```python
from build123d import *

# Parameters (mm, degrees)
SKETCH1_R                        = 39.7891
SKETCH1_R_2                      = 38.1635
BOSS_EXTRUDE1_DEPTH              = 411.48
CUT_EXTRUDE1_START               = -1.66704
SKETCH2_R                        = 1.778
CUT_EXTRUDE1_DEPTH               = 1.66704
CIRPATTERN1_COUNT                = 3
PRESSURE_START                   = -1.699963
SKETCH3_R                        = 2.38125
PRESSURE_EQUALIZATION_HOLE_DEPTH = 1.699963
CIRPATTERN2_COUNT                = 3
SKETCH4_R                        = 1.7859375
CUT_EXTRUDE3_DEPTH               = 1.667411
CIRPATTERN3_COUNT                = 3


with BuildPart() as part:
    # Sketch1 → Boss-Extrude1 (new body)
    with BuildSketch(Plane(origin=(0, 0, 0), x_dir=(1, 0, 0), z_dir=(0, 1, 0))):
        Circle(SKETCH1_R)
        Circle(SKETCH1_R_2, mode=Mode.SUBTRACT)
    extrude(amount=BOSS_EXTRUDE1_DEPTH)

    # Sketch2 → Cut-Extrude1 (cut)
    with BuildSketch(Plane(origin=(-19.89455, 0, 34.458371394), x_dir=(0, -1, 0), z_dir=(-0.5, 0, 0.866025404)).offset(CUT_EXTRUDE1_START)):
        with Locations((-76.2, 0)):
            Circle(SKETCH2_R)
    cut_extrude1 = extrude(amount=CUT_EXTRUDE1_DEPTH, mode=Mode.SUBTRACT)

    # CirPattern1: Cut-Extrude1 ×3 about axis
    cirpattern1_axis = Axis((0, -7.62, 0), (0, 1, 0))
    for i in range(1, CIRPATTERN1_COUNT):
        add(cut_extrude1.rotate(cirpattern1_axis, i * 360 / CIRPATTERN1_COUNT), mode=Mode.SUBTRACT)

    # Sketch3 → Pressure Equalization Hole (cut)
    with BuildSketch(Plane(origin=(-19.89455, 0, 34.458371394), x_dir=(0, -1, 0), z_dir=(-0.5, 0, 0.866025404)).offset(PRESSURE_START)):
        with Locations((-205.74, 0)):
            Circle(SKETCH3_R)
    pressure_equalization_hole = extrude(amount=PRESSURE_EQUALIZATION_HOLE_DEPTH, mode=Mode.SUBTRACT)

    # CirPattern2: Pressure Equalization Hole ×3 about axis
    cirpattern2_axis = Axis((0, -7.62, 0), (0, 1, 0))
    for i in range(1, CIRPATTERN2_COUNT):
        add(pressure_equalization_hole.rotate(cirpattern2_axis, i * 360 / CIRPATTERN2_COUNT), mode=Mode.SUBTRACT)

    # Sketch4 → Cut-Extrude3 (cut)
    with BuildSketch(Plane(origin=(39.7891, 0, 0), x_dir=(0, -1, 0), z_dir=(-1, 0, 0))):
        with Locations((-377.6726, 0)):
            Circle(SKETCH4_R)
    cut_extrude3 = extrude(amount=CUT_EXTRUDE3_DEPTH, mode=Mode.SUBTRACT)

    # CirPattern3: Cut-Extrude3 ×3 about axis
    cirpattern3_axis = Axis((0, -7.62, 0), (0, 1, 0))
    for i in range(1, CIRPATTERN3_COUNT):
        add(cut_extrude3.rotate(cirpattern3_axis, i * 360 / CIRPATTERN3_COUNT), mode=Mode.SUBTRACT)


solid = part.part
```
CAD build for the part. Positions are in the model's coordinates, mm. Give positions to 0.01 mm unless a question says otherwise; leave off trailing zeros. Loops run counter-clockwise (first coordinate to the right, second up) from the corner with the lowest first, then second, coordinate; pieces in that order, holes last. Notation, with made-up numbers: (67, -22.75) -> (119, -22.75) arc R9 cw to (119, -7.75) -> close; hole circle Ø7 at (2.5, -17.75). An arc over 180 degrees is marked (long way). Use a Markdown table: item, result.
1. Slice it at B-B (z = -13). List the corners of the cut face in (x, y), plus the area to 3 significant figures.
Check result:
| item | result |
|---|---|
| outline | (-37.61, 0) -> (-35.88, 0) -> (-35.88, 411.48) -> (-37.61, 411.48) -> close; (35.88, 0) -> (37.61, 0) -> (37.61, 411.48) -> (35.88, 411.48) -> close |
| area | 1,420 mm^2 |
2. Wall check: L1, parallel to Y at x = 38.95, z = 0; L2, parallel to Z at x = 0, y = 110.5. Give the ranges that are in metal, low to high. Write a range as [from, to].
Check result:
| item | result |
|---|---|
| L1 | y = [0, 74.42], [77.98, 203.36], [208.12, 375.89], [379.46, 411.48] |
| L2 | z = [-39.79, -38.16], [38.16, 39.79] |
3. Slice it at C-C (y = 132). List the corners of the cut face in (x, z).
Check result:
| item | result |
|---|---|
| outline | circle Ø79.58 at (0, 0); hole circle Ø76.33 at (0, 0) |
4. Slice it at A-A (x = 0). List the corners of the cut face in (y, z).
Check result:
| item | result |
|---|---|
| outline | (0, -39.79) -> (411.48, -39.79) -> (411.48, -38.16) -> (0, -38.16) -> close; (0, 38.16) -> (411.48, 38.16) -> (411.48, 39.79) -> (0, 39.79) -> close |
5. Flat gauge pins, fed straight in: pin 1 (1.5 mm diameter, centred on y = 327.5, z = 15, fed in from -X); pin 2 (8 mm diameter, centred on y = 184.5, z = 11.5, fed in from +X); pin 3 (2 mm diameter, centred on y = 301.5, z = -10, fed in from +X). Where does each tip first touch, or does it go through?
Check result:
| item | result |
|---|---|
| pin 1 | stops at x = -37.15 |
| pin 2 | stops at x = 39.08 |
| pin 3 | stops at x = 38.76 |
6. Mould opens along X. For faces 1 (the cylindrical face through (-5.18, 202.86, -39.45)), 2 (the cylindrical face through (20.516, 202.86, -32.18)) say: pulls with the +X half, pulls with the -X half, needs draft (parallel to the pull), parting line crosses it, or undercut.
Check result:
| item | result |
|---|---|
| face 1 | parting line crosses it |
| face 2 | undercut |
